from build123d import *

# Parameters (mm, degrees)
F0_W     = 6.4389
F0_H     = 25.5778
F0_W_2   = 25.5778
F0_H_2   = 6.4389
F1_DEPTH = 6.35


with BuildPart() as f1:
    # F0 (on Right) → F1 (new body)
    with BuildSketch(Plane.YZ):
        Polygon((0, 25.3111), (0, 0), (18.9611, 0), (44.5389, 0), (69.7611, 0), (95.3389, 0), (114.3, 0), (114.3, 25.3111), (114.3, 50.8889), (114.3, 76.2), (0, 76.2), (0, 50.8889), align=None)
        with Locations((-3.21945, 38.1)):
            Rectangle(F0_W, F0_H)
        with Locations((31.75, -3.21945)):
            Rectangle(F0_W_2, F0_H_2)
        with Locations((82.55, -3.21945)):
            Rectangle(F0_W_2, F0_H_2)
        with Locations((117.51945, 38.1)):
            Rectangle(F0_W, F0_H)
    extrude(amount=F1_DEPTH)


solid = f1.part
Can you work these out from the model? Positions are in its coordinate system, mm. A direction names the side the tool comes from. Give positions to 0.01 mm unless a question says otherwise; leave off trailing zeros. Order: outer loops, then holes, each group sorted by start corner. A loop starts at its lowest first (then second) coordinate and runs counter-clockwise, first axis right, second up. Notation, with made-up numbers: M 54.25,-32.5 L 64.25,-32.5 A6 cw 64.25,-22.5 Z; hole C -7.75,-23.5 d9. An arc over 180 degrees is marked long. Use one line per item in the form item = value.
Item 1: If we section it at A-A, the plane x = 3.5: Write out the boundary of the cut face in (y, z), and give its area (3 significant figures).
Values follow:
outline = M -6.44,25.31 L 0,25.31 L 0,0 L 18.96,0 L 18.96,-6.44 L 44.54,-6.44 L 44.54,0 L 69.76,0 L 69.76,-6.44 L 95.34,-6.44 L 95.34,0 L 114.3,0 L 114.3,25.31 L 120.74,25.31 L 120.74,50.89 L 114.3,50.89 L 114.3,76.2 L 0,76.2 L 0,50.89 L -6.44,50.89 Z
area = 9,370 mm^2
Item 2: For faces 1 (the flat face through (3, 120.739, 38)), 2 (the flat face through (3, 82, -6.439)), 3 (the flat face through (3, 18.961, -3)), 4 (the flat face through (3, 114.3, 12)), 5 (the flat face through (3, 114.3, 63)), which set-ups out of +Z, -Z, +X, -X, +Y, -Y let a thin tool reach every point of the face, with its end or its side?
Values follow:
face_1 = +Z, -Z, +X, -X, +Y
face_2 = -Z, +X, -X, +Y, -Y
face_3 = -Z, +X, -X, -Y
face_4 = -Z, +X, -X, +Y
face_5 = +Z, +X, -X, +Y
Item 3: Thinking about a two-plate mould opening in Y: for faces 6 (the flat face through (3, 95.339, -3)), 7 (the flat face through (3, 69.761, -3)), 8 (the flat face through (3, 0, 64)), 9 (the flat face through (3, 57, 0)), which applies, pulls with the +Y half, pulls with the -Y half, needs draft (parallel to the pull), parting line crosses it, or undercut?
Values follow:
face_6 = pulls with the +Y half
face_7 = undercut
face_8 = pulls with the -Y half
face_9 = undercut
Item 4: Will these pins go through, and if not, where does the flat tip stop? pin 1 Ø1.9 at (x, z) = (4, 65.5) entering from +Y; pin 2 Ø1.9 at (x, z) = (2, -4.5) entering from -Y; pin 3 Ø3 at (x, z) = (4, 65.5) entering from -Y.
Values follow:
pin_1 = 114.3
pin_2 = 18.96
pin_3 = 0
Item 5: If we section it at C-C, the plane z = 13.5: Write out the boundary of the cut face in (x, y), and give its area (3 significant figures).
Values follow:
outline = M 0,0 L 6.35,0 L 6.35,114.3 L 0,114.3 Z
area = 726 mm^2
Item 6: If we section it at B-B, the plane y = 54: Write out the boundary of the cut face in (x, z).
Values follow:
outline = M 0,0 L 6.35,0 L 6.35,76.2 L 0,76.2 Z
Item 7: If I drill on line 1 along Z through (x, y) = (3.5, 59); line 2 along Y through (x, z) = (2.5, -1); line 3 along Y through (x, z) = (2.5, 63), over which ranges is the centre line in solid material (lowest first)? Write a range as [from, to].
Values follow:
line_1 = [0, 76.2]
line_2 = [18.96, 44.54], [69.76, 95.34]
line_3 = [0, 114.3]
